Source: CAD feature listing. Evaluate the final solid. Frame: model axes, mm. Face numbers are marked on the shaded views. A direction names the side the tool comes from. Coordinates: 2 decimals unless noted, no trailing zeros. Order: outer loops, then holes, each group sorted by start corner. A loop starts at its lowest first (then second) coordinate and runs counter-clockwise, first axis right, second up. Notation, with made-up numbers: (18.5, 45.25) -> (69.5, 45.25) arc R25 cw to (69.5, 64.25) -> close; hole circle Ø11 at (71.25, -19.5). An arc over 180 degrees is marked (long way). Put each result on its own line as item: value.
from build123d import *

# Parameters (mm, degrees)
SKETCH_1_W           = 60
SKETCH_1_H           = 34
EXTRUDE_1_DEPTH      = 6
CUT_EXTRUDE_1_DEPTH  = 7
EXTRUDE_2_DEPTH      = 6
SKETCH_3_R           = 2.1
SKETCH_3_W           = 7
SKETCH_3_H           = 6
CUT_EXTRUDE_11_DEPTH = 7
EXTRUDE_21_DEPTH     = 6
SKETCH_31_R          = 2.1
SKETCH_31_W          = 7
SKETCH_31_H          = 6
CUT_EXTRUDE_12_DEPTH = 7


with BuildPart() as part:
    # Эскиз1 → Бобышка-Вытянуть1 (new body)
    with BuildSketch(Plane.XY):
        with Locations((4.02043073, 14.078379342)):
            Rectangle(SKETCH_1_W, SKETCH_1_H)
    extrude(amount=EXTRUDE_1_DEPTH)

    # Эскиз2 → Вырез-Вытянуть1 (cut, through all)
    with BuildSketch(Plane.XY.offset(6)):
        with BuildLine():
            Line((-2.02956927, -2.921620658), (-2.02956927, 5.078379342))
            ThreePointArc((-2.02956927, 5.078379342), (4.02043073, 11.128379342), (10.07043073, 5.078379342))
            Line((10.07043073, 5.078379342), (10.07043073, -2.921620658))
            ThreePointArc((10.07043073, -2.921620658), (4.02043073, -8.971620658), (-2.02956927, -2.921620658))
        make_face()
    extrude(amount=-CUT_EXTRUDE_1_DEPTH, mode=Mode.SUBTRACT)

    # Эскиз21 → Бобышка-Вытянуть2 (add)
    with BuildSketch(Plane(origin=(24.02043073, 14.078379342, 6), x_dir=(0, -1, 0), z_dir=(0, 0, -1))):
        with BuildLine():
            Line((13, 53), (-13, 53))
            ThreePointArc((-13, 53), (-14.118033989, 52.736067977), (-15, 52))
            Line((-15, 52), (-16.2, 50.4))
            ThreePointArc((-16.2, 50.4), (-16.552786405, 50.105572809), (-17, 50))
            Line((-17, 50), (17, 50))
            ThreePointArc((17, 50), (16.552786405, 50.105572809), (16.2, 50.4))
            Line((16.2, 50.4), (15, 52))
            ThreePointArc((15, 52), (14.118033989, 52.736067977), (13, 53))
        make_face()
    extrude(amount=EXTRUDE_2_DEPTH)

    # Эскиз3 → Вырез-Вытянуть11 (cut, through all)
    with BuildSketch(Plane(origin=(24.02043073, 14.078379342, 0), x_dir=(0, -1, 0), z_dir=(0, 0, -1))):
        with Locations((0, 47)):
            Circle(SKETCH_3_R)
        with Locations((9.531849908, 47)):
            Rectangle(SKETCH_3_W, SKETCH_3_H)
        with Locations((-9.531849908, 47)):
            Rectangle(SKETCH_3_W, SKETCH_3_H)
    extrude(amount=-CUT_EXTRUDE_11_DEPTH, mode=Mode.SUBTRACT)

    # Эскиз22 → Бобышка-Вытянуть21 (add)
    with BuildSketch(Plane(origin=(-15.97956927, 14.078379342, 6), x_dir=(0, 1, 0), z_dir=(0, 0, -1))):
        with BuildLine():
            Line((13, 53), (-13, 53))
            ThreePointArc((-13, 53), (-14.118033989, 52.736067977), (-15, 52))
            Line((-15, 52), (-16.2, 50.4))
            ThreePointArc((-16.2, 50.4), (-16.552786405, 50.105572809), (-17, 50))
            Line((-17, 50), (17, 50))
            ThreePointArc((17, 50), (16.552786405, 50.105572809), (16.2, 50.4))
            Line((16.2, 50.4), (15, 52))
            ThreePointArc((15, 52), (14.118033989, 52.736067977), (13, 53))
        make_face()
    extrude(amount=EXTRUDE_21_DEPTH)

    # Эскиз31 → Вырез-Вытянуть12 (cut, through all)
    with BuildSketch(Plane(origin=(-15.97956927, 14.078379342, 0), x_dir=(0, 1, 0), z_dir=(0, 0, -1))):
        with Locations((0, 47)):
            Circle(SKETCH_31_R)
        with Locations((9.531849908, 47)):
            Rectangle(SKETCH_31_W, SKETCH_31_H)
        with Locations((-9.531849908, 47)):
            Rectangle(SKETCH_31_W, SKETCH_31_H)
    extrude(amount=-CUT_EXTRUDE_12_DEPTH, mode=Mode.SUBTRACT)


solid = part.part
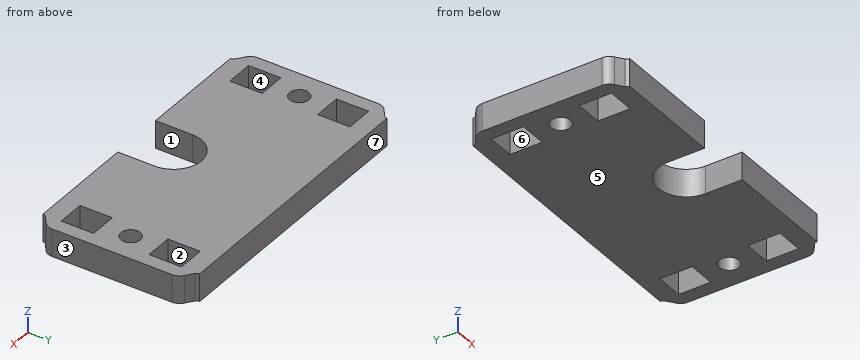
1. Ray query, line 1 along Y through (x, z) = (-25.5, 4.1); line 2 along X through (y, z) = (21, 4.05); line 3 along Y through (x, z) = (-23, 2.8). Return the intervals inside material, ascending.
Numbers:
line 1: y = -2.92 to 1.05, 8.05 to 20.11, 27.11 to 31.08
line 2: x = -28.98 to -25.98, -19.98 to 28.02, 34.02 to 37.02
line 3: y = -2.92 to 1.05, 8.05 to 11.98, 16.18 to 20.11, 27.11 to 31.08
2. Cut plane B-B on y = 21.5. Output: boundary loops of the cut face in (x, z), plus the area to 3 significant figures.
Numbers:
outline: (-28.98, 0) -> (-25.98, 0) -> (-25.98, 6) -> (-28.98, 6) -> close; (-19.98, 0) -> (28.02, 0) -> (28.02, 6) -> (-19.98, 6) -> close; (34.02, 0) -> (37.02, 0) -> (37.02, 6) -> (34.02, 6) -> close
area: 324 mm2
3. Set-up query: the marked faces 1, 2 and 3. Return all of +Z, -Z, +X, -X, +Y, -Y with unobstructed straight access to the full face (end or side cutting, diameter ignored); none if empty.
Numbers:
face 1: +Z, -Z, -Y
face 2: +Z, -Z
face 3: +Z, -Z, +X, +Y, -Y
4. First-contact query: pin 1 (4 mm diameter, centred on x = -22.98, y = 14.08, fed in from +Z). Flat tip, straight axial feed; report the tip coordinate or a pass-through.
Numbers:
pin 1: passes through
5. Cut plane C-C on x = 9. Output: boundary loops of the cut face in (y, z), plus the area to 3 significant figures.
Numbers:
outline: (8.51, 0) -> (31.08, 0) -> (31.08, 6) -> (8.51, 6) -> close
area: 135 mm2
6. Cut plane D-D on z = 4.1. Count the separate pieces of the cut face and the enclosed holes in it, plus the area to 3 significant figures.
Numbers:
separate pieces: 1
enclosed holes: 6
area: 1,870 mm2
7. Cut plane A-A on y = 3. Output: boundary loops of the cut face in (x, z).
Numbers:
outline: (-28.98, 0) -> (-25.98, 0) -> (-25.98, 6) -> (-28.98, 6) -> close; (-19.98, 0) -> (-2.03, 0) -> (-2.03, 6) -> (-19.98, 6) -> close; (10.07, 0) -> (28.02, 0) -> (28.02, 6) -> (10.07, 6) -> close; (34.02, 0) -> (37.02, 0) -> (37.02, 6) -> (34.02, 6) -> close
8. Pull-direction query (Y, two-part tool) for the marked faces 4, 5, 6 and 7; classes: pulls with the +Y half, pulls with the -Y half, needs draft (parallel to the pull), parting line crosses it, or undercut.
Numbers:
face 4: undercut
face 5: needs draft
face 6: undercut
face 7: pulls with the +Y half
